from build123d import *

# Parameters (mm, degrees)
EXTRUDE_1_DEPTH         = 37
SHELL_1_T               = -12
HOLE_WIZARD_M5_2_D      = 5.5
HOLE_WIZARD_M5_1_REACH  = 680.344
HOLE_WIZARD_M5_1_BORE_R = 2.75


with BuildPart() as part:
    # 草图1 → 拉伸-薄壁1 (new, symmetric)
    with BuildSketch(Plane.XY):
        with BuildLine():
            Line((0, -27.5), (500, -27.5))
            ThreePointArc((500, -27.5), (627.5, 100), (500, 227.5))
            Line((500, 227.5), (300, 227.5))
            Line((300, 227.5), (300, 172.5))
            Line((300, 172.5), (500, 172.5))
            ThreePointArc((500, 172.5), (572.5, 100), (500, 27.5))
            Line((500, 27.5), (0, 27.5))
            Line((0, 27.5), (0, -27.5))
        make_face()
    extrude(amount=EXTRUDE_1_DEPTH, both=True)

    # 抽壳1
    shell_1_openings = [part.faces().sort_by_distance(p)[0] for p in [
        (0, 0, 0),
        (300, 200, 0),
    ]]
    offset(amount=SHELL_1_T, openings=shell_1_openings, kind=Kind.INTERSECTION)

    # M5 间隙孔2 (through all)
    with Locations(Plane(origin=(0, 27.5, 0), x_dir=(1, 0, 0), z_dir=(0, 1, 0))):
        with Locations((12, 32.5), (34.5, 32.5), (34.5, -32.5), (12, -32.5)):
            Hole(HOLE_WIZARD_M5_2_D / 2)

    # M5 间隙孔1 bore → M5 间隙孔1 (cut, up to next)
    with BuildSketch(Plane(origin=(0, 227.5, 0), x_dir=(1, 0, 0), z_dir=(0, 1, 0)), mode=Mode.PRIVATE) as hole_wizard_m5_1_sk1:
        with Locations((313, 32.5)):
            Circle(HOLE_WIZARD_M5_1_BORE_R)
    hole_wizard_m5_1_tool1 = extrude(hole_wizard_m5_1_sk1.sketch, amount=-HOLE_WIZARD_M5_1_REACH, mode=Mode.PRIVATE) & part.part
    # M5 间隙孔1 bore → M5 间隙孔1 (cut, up to next)
    with BuildSketch(Plane(origin=(0, 227.5, 0), x_dir=(1, 0, 0), z_dir=(0, 1, 0)), mode=Mode.PRIVATE) as hole_wizard_m5_1_sk2:
        with Locations((335.5, 32.5)):
            Circle(HOLE_WIZARD_M5_1_BORE_R)
    hole_wizard_m5_1_tool2 = extrude(hole_wizard_m5_1_sk2.sketch, amount=-HOLE_WIZARD_M5_1_REACH, mode=Mode.PRIVATE) & part.part
    # M5 间隙孔1 bore → M5 间隙孔1 (cut, up to next)
    with BuildSketch(Plane(origin=(0, 227.5, 0), x_dir=(1, 0, 0), z_dir=(0, 1, 0)), mode=Mode.PRIVATE) as hole_wizard_m5_1_sk3:
        with Locations((335.5, -32.5)):
            Circle(HOLE_WIZARD_M5_1_BORE_R)
    hole_wizard_m5_1_tool3 = extrude(hole_wizard_m5_1_sk3.sketch, amount=-HOLE_WIZARD_M5_1_REACH, mode=Mode.PRIVATE) & part.part
    # M5 间隙孔1 bore → M5 间隙孔1 (cut, up to next)
    with BuildSketch(Plane(origin=(0, 227.5, 0), x_dir=(1, 0, 0), z_dir=(0, 1, 0)), mode=Mode.PRIVATE) as hole_wizard_m5_1_sk4:
        with Locations((313, -32.5)):
            Circle(HOLE_WIZARD_M5_1_BORE_R)
    hole_wizard_m5_1_tool4 = extrude(hole_wizard_m5_1_sk4.sketch, amount=-HOLE_WIZARD_M5_1_REACH, mode=Mode.PRIVATE) & part.part
    add(hole_wizard_m5_1_tool1.solids().sort_by_distance((313, 227.5, -32.5))[0], mode=Mode.SUBTRACT)
    add(hole_wizard_m5_1_tool2.solids().sort_by_distance((335.5, 227.5, -32.5))[0], mode=Mode.SUBTRACT)
    add(hole_wizard_m5_1_tool3.solids().sort_by_distance((335.5, 227.5, 32.5))[0], mode=Mode.SUBTRACT)
    add(hole_wizard_m5_1_tool4.solids().sort_by_distance((313, 227.5, 32.5))[0], mode=Mode.SUBTRACT)


solid = part.part
The model under review builds one solid part; all positions refer to its coordinate system, in mm. A direction names the side the tool comes from. Round coordinates to 2 decimals unless told otherwise and drop trailing zeros. Loops run counter-clockwise (first coordinate to the right, second up) from the corner with the lowest first, then second, coordinate; pieces in that order, holes last. Notation, with made-up numbers: M 61.25,-30.75 L 112.25,-30.75 A25 ccw 112.25,5.25 Z; hole C 72,85 d11. An arc over 180 degrees is marked long. Answer as a JSON object with one key per item and string values.
Item 1: Clearance check with flat-ended pins moving along their axes: P1, Ø12, axis at y = 76, z = -2.5, coming from the +X side; P2, Ø4, axis at y = 140.5, z = -28, coming from the +X side; P3, Ø4, axis at y = 125, z = 19, coming from the -X side. State where each tip first meets the part, or that it passes through.
Check sheet entries:
{"P1": "x = 626.22", "P2": "x = 621.55", "P3": "x = 567.28"}
Item 2: We need section B-B, the plane z = 13.5. State the section outline as (x, y) points.
Check sheet entries:
{"outline": "M 0,-27.5 L 500,-27.5 A127.5 ccw 500,227.5 L 300,227.5 L 300,215.5 L 500,215.5 A115.5 cw 500,-15.5 L 0,-15.5 Z; M 0,15.5 L 500,15.5 A84.5 ccw 500,184.5 L 300,184.5 L 300,172.5 L 500,172.5 A72.5 cw 500,27.5 L 0,27.5 Z"}
Item 3: We need section A-A, the plane x = 459. State the section outline as (y, z) points, and give its area (3 significant figures).
Check sheet entries:
{"outline": "M -27.5,-37 L 27.5,-37 L 27.5,37 L -27.5,37 Z; M 172.5,-37 L 227.5,-37 L 227.5,37 L 172.5,37 Z; hole M -15.5,-25 L 15.5,-25 L 15.5,25 L -15.5,25 Z; hole M 184.5,-25 L 215.5,-25 L 215.5,25 L 184.5,25 Z", "area": "5,040 mm2"}
Item 4: We need section D-D, the plane x = 143. State the section outline as (y, z) points, and give its area (3 significant figures).
Check sheet entries:
{"outline": "M -27.5,-37 L 27.5,-37 L 27.5,37 L -27.5,37 Z; hole M -15.5,-25 L 15.5,-25 L 15.5,25 L -15.5,25 Z", "area": "2,520 mm2"}
Item 5: We need section C-C, the plane y = 100. State the section outline as (x, z) points, and give its area (3 significant figures).
Check sheet entries:
{"outline": "M 572.5,-37 L 627.5,-37 L 627.5,37 L 572.5,37 Z; hole M 584.5,-25 L 615.5,-25 L 615.5,25 L 584.5,25 Z", "area": "2,520 mm2"}
Item 6: For line 1 along Y through (x, z) = (436, -18.5); line 2 along Z through (x, y) = (12, 8); line 3 along Y through (x, z) = (158, 3), list the stretches that pass through material, from the lowest coordinate up.
Check sheet entries:
{"line 1": "-27.5 to -15.5, 15.5 to 27.5, 172.5 to 184.5, 215.5 to 227.5", "line 2": "-37 to -35.25, -29.75 to -25, 25 to 29.75, 35.25 to 37", "line 3": "-27.5 to -15.5, 15.5 to 27.5"}
Item 7: The part is to be moulded in two halves that separate along Z. For faces 1 (the face through (247, -27.5, 1)), 2 (the face through (379, 17, -37)), 3 (the face through (352, 15, 25)), say which applies: +Z half, -Z half, draft (parallel to the pull), parting line (faces both ways), or undercut.
Check sheet entries:
{"face 1": "draft", "face 2": "-Z half", "face 3": "undercut"}
Item 8: Tool access review of faces 4 (the face through (584.48, 101.86, 0.35)), 5 (the face through (399, 172.5, 1)), 6 (the face through (379, 17, 37)), 7 (the face through (253, 15.5, 0)), 8 (the face through (300, 182, 1)): name each direction out of +Z, -Z, +X, -X, +Y, -Y from which nothing blocks a thin tool from reaching the whole face with its end or side.
Check sheet entries:
{"face 4": "none", "face 5": "+Z, -Z, -X", "face 6": "+Z, +X, -X, +Y, -Y", "face 7": "-X", "face 8": "+Z, -Z, -X, +Y"}
